```python
from build123d import *

# Parameters (mm, degrees)
SKETCH1_W           = 38.1
SKETCH1_H           = 12.7
BOSS_EXTRUDE1_DEPTH = 4.7498
SKETCH2_R           = 2.54
CUT_EXTRUDE1_DEPTH  = 4.7498
SKETCH4_W           = 38.1
SKETCH4_H           = 4.749919389
BOSS_EXTRUDE2_DEPTH = 14.3002
SKETCH5_R           = 3.81
BOSS_EXTRUDE3_DEPTH = 38.1


with BuildPart() as part:
    # Sketch1 → Boss-Extrude1 (new body)
    with BuildSketch(Plane(origin=(0, 0, 0), x_dir=(1, 0, 0), z_dir=(0, 1, 0))):
        with Locations((19.05, 6.35)):
            Rectangle(SKETCH1_W, SKETCH1_H)
    extrude(amount=BOSS_EXTRUDE1_DEPTH)

    # Sketch2 → Cut-Extrude1 (cut)
    with BuildSketch(Plane(origin=(0, 4.7498, 0), x_dir=(1, 0, 0), z_dir=(0, 1, 0))):
        with Locations(Location((6.35, 5.9436, 0), (0, 0, 270))):
            Circle(SKETCH2_R)
        with Locations(Location((31.75, 5.9436, 0), (0, 0, 270))):
            Circle(SKETCH2_R)
    extrude(amount=-CUT_EXTRUDE1_DEPTH, mode=Mode.SUBTRACT)

    # Sketch4 → Boss-Extrude2 (add)
    with BuildSketch(Plane.XY):
        with Locations((19.05, 2.374840306)):
            Rectangle(SKETCH4_W, SKETCH4_H)
    extrude(amount=BOSS_EXTRUDE2_DEPTH)

    # Sketch5 → Boss-Extrude3 (add)
    with BuildSketch(Plane.ZY):
        with Locations((7.1501, 8.127910458)):
            Circle(SKETCH5_R)
    extrude(amount=-BOSS_EXTRUDE3_DEPTH)


solid = part.part
```
Here's how the part is built. I have some questions about the finished solid (model axes, mm). A direction names the side the tool comes from. Give positions to 0.01 mm unless a question says otherwise; leave off trailing zeros. Write each loop counter-clockwise with the first axis right and the second up, starting at its lowest first coordinate (ties: lowest second). Pieces come first, ordered by that corner, then holes. Notation, with made-up numbers: M -17.5,21.5 L 31.5,21.5 A20 ccw 31.5,57.5 Z; hole C -3.75,-2 d2. An arc over 180 degrees is marked long. Put each result on its own line as item: value. Start each with the question number.
Item 1: Thinking about a two-plate mould opening in Y: for faces 4 (the flat face through (19, 0, 7)), 5 (the cylindrical face through (18.783, 11.935, 7.292)), 6 (the flat face through (0, 3, 4)), which applies, +Y half, -Y half, draft (parallel to the pull), parting line (faces both ways), or undercut?
Item 2: I need wall thicknesses on L1, parallel to Z at x = 5, y = 1.25; L2, parallel to Y at x = 22.5, z = 11.25; L3, parallel to Y at x = 18.5, z = 4. Which ranges of each line are inside material? Lowest first, please. Write a range as from..to.
Item 3: On a 3-axis mill with a long thin cutter (end or side, diameter ignored), from which of +Z, -Z, +X, -X, +Y, -Y can I reach the whole of each face in a straight line? I mean faces 1 (the flat face through (19, 4.75, 12)), 2 (the flat face through (19, 4.75, -4)), 3 (the flat face through (19, 0, -6)). Say none if no direction works.
Item 4: Will this pin go through, and if not, where does the flat tip stop? pin 1 (6 mm diameter, centred on x = 15.5, z = 12, fed in from +Y).
Item 5: If we section it at D-D, the plane z = -10.5: Write out the boundary of the cut face in (x, y).
Item 6: If we section it at B-B, the plane y = 3: Write out the boundary of the cut face in (x, z).
Values:
1. face 4: -Y half
1. face 5: undercut
1. face 6: draft
2. L1: -12.7..-8.1, -3.79..14.3
2. L2: 0..4.75
2. L3: 0..4.75, 5.98..10.27
3. face 1: +Z, +X, -X
3. face 2: -Z, +X, -X
3. face 3: +Z, -Z, +X, -X, -Y
4. pin 1: y = 11.46
5. outline: M 0,0 L 38.1,0 L 38.1,4.75 L 0,4.75 Z
6. outline: M 0,-12.7 L 38.1,-12.7 L 38.1,14.3 L 0,14.3 Z; hole C 6.35,-5.94 d5.08; hole C 31.75,-5.94 d5.08
